The model under review builds one solid part; all positions refer to its coordinate system, in mm. Face numbers are marked on the shaded views. Round coordinates to 2 decimals unless told otherwise and drop trailing zeros. Write each loop counter-clockwise with the first axis right and the second up, starting at its lowest first coordinate (ties: lowest second). Pieces come first, ordered by that corner, then holes.
Item 1: Add section D-D (x = -21). Give the boundary of the cut face in (y, z), plus the area to 3 significant figures.
Item 2: Clearance check with flat-ended pins moving along their axes: pin 1 Ø1.5 at (y, z) = (-14, -29.5) entering from +X; pin 2 Ø2 at (x, z) = (-14, -22) entering from -Y; pin 3 Ø6 at (x, y) = (15, -21.9) entering from +Z; pin 4 Ø2 at (x, z) = (-22.5, 0.5) entering from -Y. State where each tip first meets the part, or that it passes through.
Item 3: Draft analysis for pull direction Z (two halves, no side actions). For the marked faces 1, 2, 3 and 4, state which applies: +Z half, -Z half, draft (parallel to the pull), parting line (faces both ways), or undercut.
Item 4: Add section A-A (x = 15). Give the boundary of the cut face in (y, z), plus the area to 3 significant figures.
Item 5: To check wall thickness, follow L1, parallel to Y at x = -15, z = -32.8; L2, parallel to Y at x = -24.5, z = 0.4; L3, parallel to Z at x = 24, y = 8.5. State the ranges of each line that lie inside material, in increasing order.
Item 6: Add section C-C (y = 4.75). Give the boundary of the cut face in (x, z).
Item 7: Add section B-B (y = -1). Give the boundary of the cut face in (x, z).
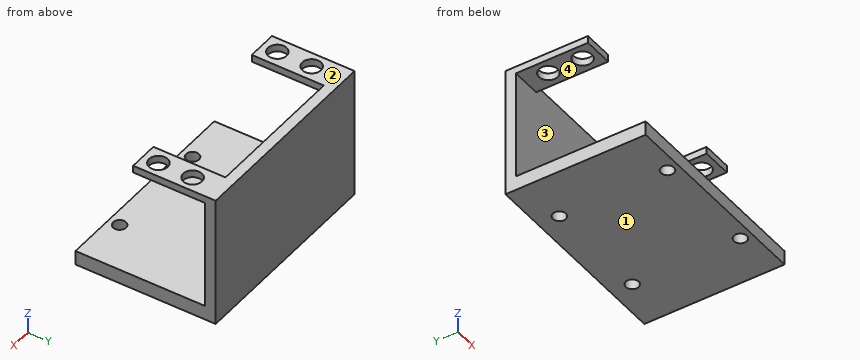
```python
from build123d import *

# Parameters (mm, degrees)
SKETCH_1_R           = 2.6
EXTRUDE_3_DEPTH      = 2
EXTRUDE_5_DEPTH      = 18.7
EXTRUDE_5_DEPTH_BACK = 2
SKETCH_9_W           = 57.159649592
SKETCH_9_H           = 11.9
EXTRUDE_6_DEPTH      = 31.5
SKETCH_10_W          = 57.159649592
SKETCH_10_H          = 11.9
EXTRUDE_7_DEPTH      = 5
SKETCH_11_W          = 57.159649592
SKETCH_11_H          = 36.5
CUT_EXTRUDE_1_DEPTH  = 10
SKETCH_12_W          = 57.159649592
SKETCH_12_H          = 4
EXTRUDE_8_DEPTH      = 35
SKETCH_13_R          = 1.8
CUT_EXTRUDE_2_DEPTH  = 10
SKETCH_14_W          = 57.159649592
SKETCH_14_H          = 36.5
EXTRUDE_9_DEPTH      = 2
CUT_EXTRUDE_3_DEPTH  = 1


with BuildPart() as part:
    # 草图1 → 凸台-拉伸3 (new body)
    # profile 1 of 2: a face of its own
    with BuildSketch(Plane.XY):
        Polygon((-28.579824796, -9), (-20.25, -9), (-20.25, 9), (-20.25, 10), (20.25, 10), (20.25, 9), (20.25, -9), (28.579824796, -9), (28.579824796, 12), (-28.579824796, 12), align=None)
        with Locations((-24.5, -4.75)):
            Circle(SKETCH_1_R, mode=Mode.SUBTRACT)
        with Locations((24.5, -4.75)):
            Circle(SKETCH_1_R, mode=Mode.SUBTRACT)
        with Locations((-24.5, 4.75)):
            Circle(SKETCH_1_R, mode=Mode.SUBTRACT)
        with Locations((24.5, 4.75)):
            Circle(SKETCH_1_R, mode=Mode.SUBTRACT)
    # profile 2 of 2: a face of its own
    with BuildSketch(Plane.XY):
        Polygon((-28.579824796, -9), (-20.25, -9), (-20.25, 9), (-20.25, 10), (20.25, 10), (20.25, 9), (20.25, -9), (28.579824796, -9), (28.579824796, 12), (-28.579824796, 12), align=None)
        with Locations((-24.5, -4.75)):
            Circle(SKETCH_1_R, mode=Mode.SUBTRACT)
        with Locations((24.5, -4.75)):
            Circle(SKETCH_1_R, mode=Mode.SUBTRACT)
        with Locations((-24.5, 4.75)):
            Circle(SKETCH_1_R, mode=Mode.SUBTRACT)
        with Locations((24.5, 4.75)):
            Circle(SKETCH_1_R, mode=Mode.SUBTRACT)
    extrude(amount=EXTRUDE_3_DEPTH)

    # 草图3 → 凸台-拉伸5 (add, two sides: drawn at the far end of the back side and taken through both)
    with BuildSketch(Plane(origin=(0, 0, 0), x_dir=(-1, 0, 0), z_dir=(0, 0, -1)).offset(-EXTRUDE_5_DEPTH_BACK)):
        Polygon((-28.579824796, 12), (-28.579824796, 10), (28.579824796, 10), (28.579824796, 12), (28.579824796, 21.9), (-28.579824796, 21.9), align=None)
    extrude(amount=EXTRUDE_5_DEPTH + EXTRUDE_5_DEPTH_BACK)

    # 草图9 → 凸台-拉伸6 (add)
    with BuildSketch(Plane.XY.offset(2)):
        with Locations((0, 15.95)):
            Rectangle(SKETCH_9_W, SKETCH_9_H)
    extrude(amount=-EXTRUDE_6_DEPTH)

    # 草图10 → 凸台-拉伸7 (add)
    with BuildSketch(Plane(origin=(0, 0, -29.5), x_dir=(-1, 0, 0), z_dir=(0, 0, -1))):
        with Locations((0, 15.95)):
            Rectangle(SKETCH_10_W, SKETCH_10_H)
    extrude(amount=EXTRUDE_7_DEPTH)

    # 草图11 → 切除-拉伸1 (cut)
    with BuildSketch(Plane(origin=(0, 21.9, 0), x_dir=(1, 0, 0), z_dir=(0, 1, 0))):
        with Locations((0, 16.25)):
            Rectangle(SKETCH_11_W, SKETCH_11_H)
    extrude(amount=-CUT_EXTRUDE_1_DEPTH, mode=Mode.SUBTRACT)

    # 草图12 → 凸台-拉伸8 (add)
    with BuildSketch(Plane.XZ.offset(-10)):
        with Locations((0, -32.5)):
            Rectangle(SKETCH_12_W, SKETCH_12_H)
    extrude(amount=EXTRUDE_8_DEPTH)

    # 草图13 → 切除-拉伸2 (cut)
    with BuildSketch(Plane(origin=(0, 0, -34.5), x_dir=(-1, 0, 0), z_dir=(0, 0, -1))):
        with Locations((-15, 8.10231344)):
            Circle(SKETCH_13_R)
        with Locations((15, -21.89768656)):
            Circle(SKETCH_13_R)
        with Locations((-15, -21.89768656)):
            Circle(SKETCH_13_R)
        with Locations((15, 8.10231344)):
            Circle(SKETCH_13_R)
    extrude(amount=-CUT_EXTRUDE_2_DEPTH, mode=Mode.SUBTRACT)

    # 草图14 → 凸台-拉伸9 (add)
    with BuildSketch(Plane(origin=(0, 11.9, 0), x_dir=(1, 0, 0), z_dir=(0, 1, 0))):
        with Locations((0, 16.25)):
            Rectangle(SKETCH_14_W, SKETCH_14_H)
    extrude(amount=EXTRUDE_9_DEPTH)

    # 草图15 → 切除-拉伸3 (cut)
    with BuildSketch(Plane.XZ.offset(-10)):
        Polygon((-28.579824796, -30.5), (28.579824796, -30.5), (28.579824796, 0), (20.25, 0), (20.25, 2), (-20.25, 2), (-20.25, 0), (-28.579824796, 0), align=None)
    extrude(amount=-CUT_EXTRUDE_3_DEPTH, mode=Mode.SUBTRACT)


solid = part.part
```
Numbers:
1. outline: (-25, -34.5) - (13.9, -34.5) - (13.9, 2) - (-9, 2) - (-9, 0) - (11, 0) - (11, -30.5) - (-25, -30.5) - close
1. area: 290 mm2
2. pin 1: passes through
2. pin 2: stops at y = 11
2. pin 3: stops at z = -30.5
2. pin 4: stops at y = -9
3. face 1: -Z half
3. face 2: +Z half
3. face 3: undercut
3. face 4: undercut
4. outline: (-25, -34.5) - (-23.7, -34.5) - (-23.7, -30.5) - (-25, -30.5) - close; (-20.1, -34.5) - (6.3, -34.5) - (6.3, -30.5) - (-20.1, -30.5) - close; (9.9, -34.5) - (13.9, -34.5) - (13.9, 2) - (11, 2) - (11, -30.5) - (9.9, -30.5) - close
4. area: 221 mm2
5. L1: y = -25 to -23.7, -20.1 to 6.3, 9.9 to 13.9
5. L2: y = -9 to -7.35, -2.15 to 2.15, 7.35 to 13.9
5. L3: z = -34.5 to -30.5, 0 to 2
6. outline: (-28.58, -34.5) - (28.58, -34.5) - (28.58, -30.5) - (-28.58, -30.5) - close; (-28.58, 0) - (-27.1, 0) - (-27.1, 2) - (-28.58, 2) - close; (-21.9, 0) - (-20.25, 0) - (-20.25, 2) - (-21.9, 2) - close; (20.25, 0) - (21.9, 0) - (21.9, 2) - (20.25, 2) - close; (27.1, 0) - (28.58, 0) - (28.58, 2) - (27.1, 2) - close
7. outline: (-28.58, -34.5) - (28.58, -34.5) - (28.58, -30.5) - (-28.58, -30.5) - close; (-28.58, 0) - (-20.25, 0) - (-20.25, 2) - (-28.58, 2) - close; (20.25, 0) - (28.58, 0) - (28.58, 2) - (20.25, 2) - close
